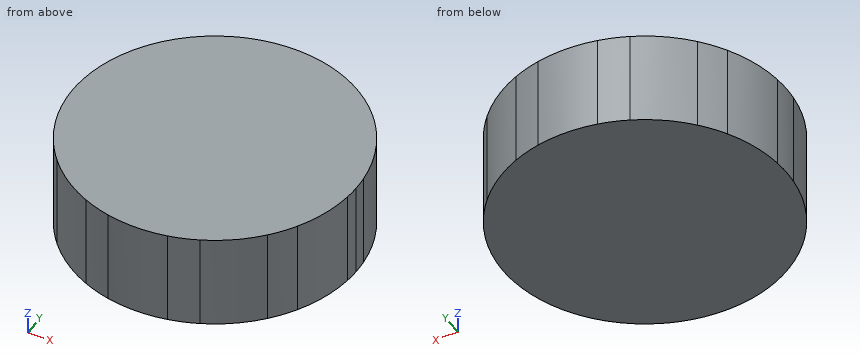
from build123d import *

# Parameters (mm, degrees)
F1_DEPTH = 25.4


# Not quite as in the source:
# - a feature names something its author has since deleted; it is built from what else it names


with BuildPart() as f1:
    # F0 (on Top) → F1 (new body)
    with BuildSketch(Plane.XY):
        with BuildLine():
            ThreePointArc((-13.8407698917, 49.932215552), (-13.693941355, 51.8586333583), (-13.6449565232, 53.7900174916))
            ThreePointArc((-13.6449565232, 53.7900174916), (-13.693941355, 55.7214016248), (-13.8407698917, 57.6478194312))
            ThreePointArc((-13.8407698917, 57.6478194312), (-15.5097032523, 65.5635649773), (-18.812266294, 72.9485120636))
            ThreePointArc((-18.812266294, 72.9485120636), (-20.9214090375, 76.1846356039), (-23.3473844667, 79.1905667238))
            ThreePointArc((-23.3473844667, 79.1905667238), (-29.3503384108, 84.6135649773), (-36.3629310228, 88.6469148221))
            ThreePointArc((-36.3629310228, 88.6469148221), (-39.9714090375, 90.0252707624), (-43.7009063693, 91.0311675426))
            ThreePointArc((-43.7009063693, 91.0311675426), (-51.7449565232, 91.8900174916), (-59.789006677, 91.0311675426))
            ThreePointArc((-59.789006677, 91.0311675426), (-63.5185040089, 90.0252707624), (-67.1269820235, 88.6469148221))
            ThreePointArc((-67.1269820235, 88.6469148221), (-74.1395746355, 84.6135649773), (-80.1425285796, 79.1905667238))
            ThreePointArc((-80.1425285796, 79.1905667238), (-82.5685040089, 76.1846356039), (-84.6776467524, 72.9485120636))
            ThreePointArc((-84.6776467524, 72.9485120636), (-87.980209794, 65.5635649773), (-89.6491431547, 57.6478194312))
            ThreePointArc((-89.6491431547, 57.6478194312), (-89.8449565232, 53.7900174916), (-89.6491431547, 49.932215552))
            ThreePointArc((-89.6491431547, 49.932215552), (-87.980209794, 42.0164700059), (-84.6776467524, 34.6315229195))
            ThreePointArc((-84.6776467524, 34.6315229195), (-82.5685040089, 31.3953993792), (-80.1425285796, 28.3894682594))
            ThreePointArc((-80.1425285796, 28.3894682594), (-74.1395746355, 22.9664700059), (-67.1269820235, 18.9331201611))
            ThreePointArc((-67.1269820235, 18.9331201611), (-63.5185040089, 17.5547642207), (-59.789006677, 16.5488674406))
            ThreePointArc((-59.789006677, 16.5488674406), (-51.7449565232, 15.6900174916), (-43.7009063693, 16.5488674406))
            ThreePointArc((-43.7009063693, 16.5488674406), (-39.9714090375, 17.5547642207), (-36.3629310228, 18.9331201611))
            ThreePointArc((-36.3629310228, 18.9331201611), (-29.3503384108, 22.9664700059), (-23.3473844667, 28.3894682594))
            ThreePointArc((-23.3473844667, 28.3894682594), (-20.9214090375, 31.3953993792), (-18.812266294, 34.6315229195))
            ThreePointArc((-18.812266294, 34.6315229195), (-15.5097032523, 42.0164700059), (-13.8407698917, 49.932215552))
        make_face()
    extrude(amount=F1_DEPTH)


solid = f1.part
Part model, mm, in its own coordinate system. Give positions to 0.01 mm unless a question says otherwise; leave off trailing zeros. Order: outer loops, then holes, each group sorted by start corner. A loop starts at its lowest first (then second) coordinate and runs counter-clockwise, first axis right, second up. Notation, with made-up numbers: (-18, 47) -> (16, 47) arc R24 ccw to (16, 83) -> close; hole circle Ø4 at (22.25, -6). An arc over 180 degrees is marked (long way). Use one line per item in the form item = value.
(1) Saw through at C-C (y = 42). Write the cut outline in (x, z), then the cut area to 3 significant figures.
Solution:
outline = (-87.97, 0) -> (-15.52, 0) -> (-15.52, 25.4) -> (-87.97, 25.4) -> close
area = 1,840 mm²
(2) Saw through at A-A (z = 21.75). Write the cut outline in (x, y).
Solution:
outline = circle Ø76.2 at (-51.74, 53.79)
(3) Drill centre lines: line 1 (Y direction, x = -51, z = 6.75); line 2 (Y direction, x = -69.5, z = 13); line 3 (X direction, y = 49, z = 12.5). Where is each one in solid material? Low to high. Write a range as from..to.
Solution:
line_1 = 15.7..91.88
line_2 = 20.08..87.5
line_3 = -89.54..-13.95
(4) Flat gauge pins, fed straight in: P1, Ø6, axis at x = -45.5, z = 20.5, coming from the -Y side; P2, Ø4, axis at y = 56, z = 9.5, coming from the +X side; P3, Ø3, axis at y = 47, z = 3, coming from the +X side. Where does each tip first touch, or does it go through?
Solution:
P1 = 15.83
P2 = -13.65
P3 = -14.01
(5) Saw through at B-B (x = -66). Write the cut outline in (y, z).
Solution:
outline = (18.46, 0) -> (89.12, 0) -> (89.12, 25.4) -> (18.46, 25.4) -> close
